Check sheet for the drawn part. Datum: minimum x, y, z corner. Units: mm. A direction names the side the tool comes from. Give positions to 0.01 mm unless a question says otherwise; leave off trailing zeros. Loops run counter-clockwise (first coordinate to the right, second up) from the corner with the lowest first, then second, coordinate; pieces in that order, holes last. Notation, with made-up numbers: (71, 12.5) - (75, 12.5) arc R9 cw to (75, 29.5) - close; hole circle Ø4 at (39, -17.75). An arc over 180 degrees is marked (long way). Use one line per item in the form item = value.
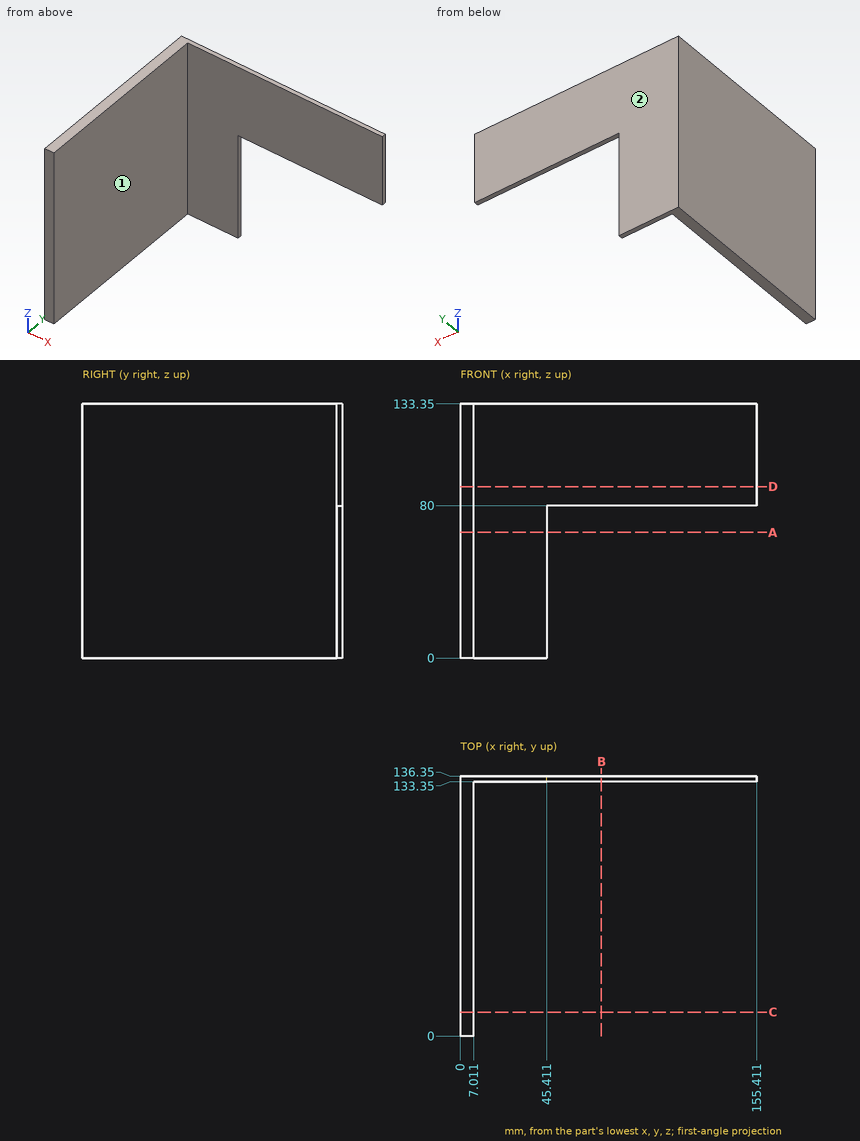
Item 1: Section check D-D on z = 90. Record the boundary of the cut face in (x, y), then the cut area to 3 significant figures.
Answer block:
outline = (0, 0) - (7.01, 0) - (7.01, 133.35) - (155.41, 133.35) - (155.41, 136.35) - (0, 136.35) - close
area = 1,400 mm2
Item 2: Access from +Z, -Z, +X, -X, +Y, -Y to the whole of each face (thin tool, end or side, straight path). Record for the marked faces 1 and 2.
Answer block:
face_1 = +Z, -Z, +X, -Y
face_2 = +Z, -Z, +X, -X, +Y
Item 3: Gauge pin test, flat ends, axial feed: P1, Ø3, axis at y = 31, z = 26, coming from the +X side; P2, Ø1.5, axis at x = 122, y = 135, coming from the -Z side; P3, Ø5, axis at x = 93, z = 110, coming from the -Y side. Record the tip position at first contact, or that the pin passes through.
Answer block:
P1 = 7.01
P2 = 80
P3 = 133.35
Item 4: Section check B-B on x = 74. Record the boundary of the cut face in (y, z), then the cut area to 3 significant figures.
Answer block:
outline = (133.35, 80) - (136.35, 80) - (136.35, 133.35) - (133.35, 133.35) - close
area = 160 mm2
Item 5: Section check A-A on z = 66. Record the boundary of the cut face in (x, y).
Answer block:
outline = (0, 0) - (7.01, 0) - (7.01, 133.35) - (45.41, 133.35) - (45.41, 136.35) - (0, 136.35) - close
Item 6: Thickness scan on L1, parallel to Y at x = 42, z = 83.5; L2, parallel to X at y = 119, z = 38. Record the ranges inside material, lowest first.
Answer block:
L1 = 133.35 to 136.35
L2 = 0 to 7.01
Item 7: Section check C-C on y = 12.5. Record the boundary of the cut face in (x, z), then the cut area to 3 significant figures.
Answer block:
outline = (0, 0) - (7.01, 0) - (7.01, 133.35) - (0, 133.35) - close
area = 935 mm2
